Here's how the part is built. I have some questions about the finished solid (model axes, mm). A direction names the side the tool comes from. Give positions to 0.01 mm unless a question says otherwise; leave off trailing zeros. Order: outer loops, then holes, each group sorted by start corner. A loop starts at its lowest first (then second) coordinate and runs counter-clockwise, first axis right, second up.
from build123d import *

# Parameters (mm, degrees)
BOSS_EXTRUDE1_DEPTH = 1940
FILLET1_R           = 3
SKETCH2_W           = 90
SKETCH2_H           = 35
CUT_EXTRUDE1_DEPTH  = 6
SKETCH3_W           = 30
SKETCH3_H           = 30
CUT_EXTRUDE2_DEPTH  = 6


with BuildPart() as part:
    # Sketch1 → Boss-Extrude1 (new body)
    with BuildSketch(Plane.XY):
        Polygon((0, 0), (87, 0), (87, -38), (117, -38), (117, -35), (90, -35), (90, 3), (0, 3), align=None)
    extrude(amount=BOSS_EXTRUDE1_DEPTH)

    # Fillet1
    fillet1_edges = [part.edges().sort_by_distance(p)[0] for p in [
        (90, 3, 970),
        (90, -35, 970),
        (87, -38, 970),
        (87, 0, 970),
    ]]
    fillet(fillet1_edges, radius=FILLET1_R)

    # Sketch2 → Cut-Extrude1 (cut)
    with BuildSketch(Plane(origin=(0, 3, 0), x_dir=(1, 0, 0), z_dir=(0, 1, 0))):
        with Locations((45, -17.5)):
            Rectangle(SKETCH2_W, SKETCH2_H)
    extrude(amount=-CUT_EXTRUDE1_DEPTH, mode=Mode.SUBTRACT)

    # Sketch3 → Cut-Extrude2 (cut)
    with BuildSketch(Plane.XZ.offset(38)):
        with Locations((102, 1925)):
            Rectangle(SKETCH3_W, SKETCH3_H)
    extrude(amount=-CUT_EXTRUDE2_DEPTH, mode=Mode.SUBTRACT)


solid = part.part
Q1. If we section it at B-B on x = 25.5: List the corners of the cut face in (y, z) for me.
Filled sheet:
outline: (0, 35) - (3, 35) - (3, 1940) - (0, 1940) - close
Q2. If we section it at C-C on y = -19: List the corners of the cut face in (x, z) for me.
Filled sheet:
outline: (87, 0) - (90, 0) - (90, 1940) - (87, 1940) - close
Q3. I'm going to push flat-ended pins straight in: P1, Ø6.5, axis at x = 53.5, y = -1, coming from the -Z side; P2, Ø1.5, axis at x = 88.5, z = 1919, coming from the -Y side; P3, Ø7, axis at x = 106, z = 1362, coming from the +Y side. Where does each tip first touch, or does it pass through?
Filled sheet:
P1: stops at z = 35
P2: stops at y = -32
P3: stops at y = -35
Q4. I need wall thicknesses on L1, parallel to Y at x = 20, z = 1199; L2, parallel to X at y = -17, z = 1560; L3, parallel to Y at x = 110, z = 384. Which ranges of each line are inside material? Lowest first, please.
Filled sheet:
L1: y = 0 to 3
L2: x = 87 to 90
L3: y = -38 to -35
Q5. If we section it at A-A on z = 403: List the corners of the cut face in (x, y) for me, plus the area to 3 significant figures.
Filled sheet:
outline: (0, 0) - (84, 0) arc R3 cw to (87, -3) - (87, -35) arc R3 ccw to (90, -38) - (117, -38) - (117, -35) - (93, -35) arc R3 cw to (90, -32) - (90, 0) arc R3 ccw to (87, 3) - (0, 3) - close
area: 465 mm2
Q6. For faces 1 (the face through (58, 1, 1940)), 2 (the face through (87, -19, 956)), 3 (the face through (90, -16, 956)), which set-ups out of +Z, -Z, +X, -X, +Y, -Y let a thin tool reach every point of the face, with its end or its side?
Filled sheet:
face 1: +Z, +X, -X, +Y, -Y
face 2: +Z, -Z, -X, -Y
face 3: +Z, -Z, +X, +Y
